Geometry: final body of the model. Coordinates: model frame, mm. A direction names the side the tool comes from. Give positions to 0.01 mm unless a question says otherwise; leave off trailing zeros. Loops run counter-clockwise (first coordinate to the right, second up) from the corner with the lowest first, then second, coordinate; pieces in that order, holes last.
from build123d import *

# Parameters (mm, degrees)
F0_W          = 90.0792330503
F0_H          = 114.4249662757
F1_DEPTH      = 50.8
F2_R          = 6.4323639035
F3_DEPTH      = 50.8
F3_DEPTH_BACK = 25.4


with BuildPart() as f1:
    # F0 (on Front) → F1 (new body)
    with BuildSketch(Plane.XZ):
        with Locations((1.1534392834, -0.5476027727)):
            Rectangle(F0_W, F0_H)
    extrude(amount=F1_DEPTH)

    # F2 (on Front) → F3 (cut, two sides)
    with BuildSketch(Plane.XZ) as f3_sk:
        with Locations((0, 27.8135836124)):
            Circle(F2_R)
        Circle(F2_R)
        with Locations((0, -29.0388520807)):
            Circle(F2_R)
    extrude(amount=-F3_DEPTH, mode=Mode.SUBTRACT)
    extrude(f3_sk.sketch, amount=F3_DEPTH_BACK, mode=Mode.SUBTRACT)


solid = f1.part
Item 1: Pin query (flat end, axial travel): pin 1 (4 mm diameter, centred on x = 2, z = -30, fed in from +Y). Return the tip coordinate at first contact, or that it passes through.
Values follow:
pin 1: stops at y = -25.4
Item 2: Section query C-C on y = -17. Return loops of the section in (x, z), plus the area to 3 significant figures.
Values follow:
outline: (-43.89, -57.76) - (46.19, -57.76) - (46.19, 56.66) - (-43.89, 56.66) - close; hole circle Ø12.86 at (0, -29.04); hole circle Ø12.86 at (0, 0); hole circle Ø12.86 at (0, 27.81)
area: 9,920 mm2
Item 3: Section query B-B on z = 0. Return loops of the section in (x, y), plus the area to 3 significant figures.
Values follow:
outline: (-43.89, -50.8) - (46.19, -50.8) - (46.19, 0) - (6.43, 0) - (6.43, -25.4) - (-6.43, -25.4) - (-6.43, 0) - (-43.89, 0) - close
area: 4,250 mm2
Item 4: Draft query along X for faces 1 (the face through (-1.394, -12.522, 21.534)), 2 (the face through (46.193, -25, -1)), 3 (the face through (-9, 0, 0)), 4 (the face through (0, -25.4, 0)). Return one class per face: +X half, -X half, draft (parallel to the pull), parting line (faces both ways), or undercut.
Values follow:
face 1: undercut
face 2: +X half
face 3: draft
face 4: undercut
Item 5: Set-up query: faces 5 (the face through (-43.886, -25, -1)), 6 (the face through (-0.84, -12.52, -22.66)). Return all of +Z, -Z, +X, -X, +Y, -Y with unobstructed straight access to the full face (end or side cutting, diameter ignored); none if empty.
Values follow:
face 5: +Z, -Z, -X, +Y, -Y
face 6: +Y
Item 6: Section query A-A on x = 0. Return loops of the section in (y, z), plus the area to 3 significant figures.
Values follow:
outline: (-50.8, -57.76) - (0, -57.76) - (0, -35.47) - (-25.4, -35.47) - (-25.4, -22.61) - (0, -22.61) - (0, -6.43) - (-25.4, -6.43) - (-25.4, 6.43) - (0, 6.43) - (0, 21.38) - (-25.4, 21.38) - (-25.4, 34.25) - (0, 34.25) - (0, 56.66) - (-50.8, 56.66) - close
area: 4,830 mm2
Item 7: Ray query, probe 1 along Z at (x, y) = (0, -10.5); probe 2 along X at (y, z) = (-16.5, 1.5); probe 3 along X at (y, z) = (-4, -31). Return the intervals inside material, ascending.
Values follow:
probe 1: z = -57.76 to -35.47, -22.61 to -6.43, 6.43 to 21.38, 34.25 to 56.66
probe 2: x = -43.89 to -6.26, 6.26 to 46.19
probe 3: x = -43.89 to -6.13, 6.13 to 46.19
